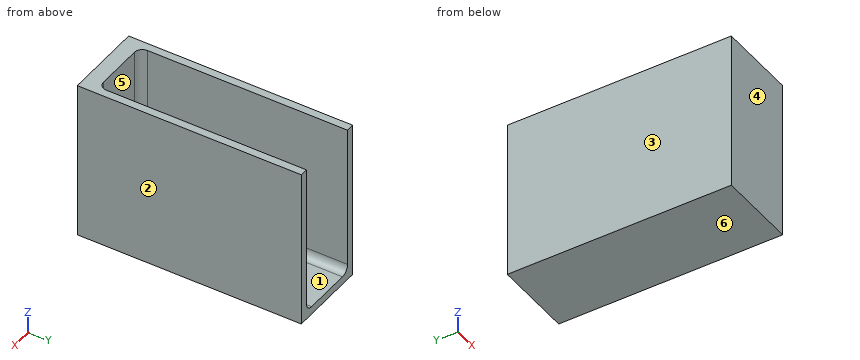
```python
from build123d import *

# Parameters (mm, degrees)
SKETCH1_W           = 25.4
SKETCH1_H           = 50.8
BOSS_EXTRUDE1_DEPTH = 5.08
BOSS_EXTRUDE2_DEPTH = 66.04
FILLET1_R           = 2.54


with BuildPart() as part:
    # Sketch1 → Boss-Extrude1 (new body)
    with BuildSketch(Plane(origin=(0, 0, 0), x_dir=(1, 0, 0), z_dir=(0, 1, 0))):
        Rectangle(SKETCH1_W, SKETCH1_H)
    extrude(amount=BOSS_EXTRUDE1_DEPTH)

    # Sketch2 → Boss-Extrude2 (add)
    with BuildSketch(Plane(origin=(0, 5.08, 0), x_dir=(1, 0, 0), z_dir=(0, 1, 0))):
        Polygon((-12.7, -25.4), (-12.7, 25.4), (12.7, 25.4), (12.7, -25.4), (10.16, -25.4), (10.16, 22.86), (-10.16, 22.86), (-10.16, -25.4), align=None)
    extrude(amount=BOSS_EXTRUDE2_DEPTH)

    # Fillet1
    fillet1_edges = [part.edges().sort_by_distance(p)[0] for p in [
        (-10.16, 5.08, 1.27),
        (0, 5.08, -22.86),
        (-10.16, 38.1, -22.86),
        (10.16, 5.08, 1.27),
        (10.16, 38.1, -22.86),
    ]]
    fillet(fillet1_edges, radius=FILLET1_R)


solid = part.part
```
Verification items for the finished model (mm, model axes). Face numbers are marked on the shaded views. A direction names the side the tool comes from. Coordinates: 2 decimals unless noted, no trailing zeros. Write each loop counter-clockwise with the first axis right and the second up, starting at its lowest first coordinate (ties: lowest second). Pieces come first, ordered by that corner, then holes. Notation, with made-up numbers: M 29,45.5 L 72,45.5 A24 ccw 72,74.5 Z; hole C 3,21 d7. An arc over 180 degrees is marked long. Answer as a JSON object with one key per item and string values. Group by question number.
(1) Tool access check on the marked faces 5 and 6. Record the directions out of +Z, -Z, +X, -X, +Y, -Y that give a thin tool (end or side, any length) a straight path to the whole face; none if there is none.
(2) Cross-section at A-A, the plane y = 54. Record the cut outline in (x, z), and give its area (3 significant figures).
(3) Release check for a two-part mould opening along X. For the marked faces 1, 2, 3 and 4 record: +X half, -X half, draft (parallel to the pull), parting line (faces both ways), or undercut.
(4) Cross-section at B-B, the plane z = 15. Record the cut outline in (x, y), and give its area (3 significant figures).
(5) Gauge pin test, flat ends, axial feed: pin 1 (6 mm diameter, centred on x = -5.5, z = -15, fed in from +Y); pin 2 (1.5 mm diameter, centred on x = -2, y = 40, fed in from +Z); pin 3 (1.5 mm diameter, centred on x = 5.5, z = 8.5, fed in from +Y). Record the tip position at first contact, or that the pin passes through.
(6) Cross-section at C-C, the plane x = -5.5. Record the cut outline in (y, z).
(7) Material ranges on line 1 (X direction, y = 31.5, z = -5.5); line 2 (Z direction, x = 6.5, y = 45); line 3 (Y direction, x = 0, z = 8), recorded low to high.
Reply:
{
 "1": {"face 5": "+Z, +Y", "face 6": "-Z, +X, -X, +Y, -Y"},
 "2": {"outline": "M -12.7,-25.4 L 12.7,-25.4 L 12.7,25.4 L 10.16,25.4 L 10.16,-20.32 A2.54 cw 7.62,-22.86 L -7.62,-22.86 A2.54 cw -10.16,-20.32 L -10.16,25.4 L -12.7,25.4 Z", "area": "312 mm²"},
 "3": {"face 1": "undercut", "face 2": "+X half", "face 3": "-X half", "face 4": "draft"},
 "4": {"outline": "M -12.7,0 L 12.7,0 L 12.7,71.12 L 10.16,71.12 L 10.16,7.62 A2.54 cw 7.62,5.08 L -7.62,5.08 A2.54 cw -10.16,7.62 L -10.16,71.12 L -12.7,71.12 Z", "area": "467 mm²"},
 "5": {"pin 1": "y = 5.24", "pin 2": "z = -22.86", "pin 3": "y = 5.08"},
 "6": {"outline": "M 0,-25.4 L 71.12,-25.4 L 71.12,-22.86 L 7.62,-22.86 A2.54 cw 5.08,-20.32 L 5.08,25.4 L 0,25.4 Z"},
 "7": {"line 1": "-12.7 to -10.16, 10.16 to 12.7", "line 2": "-25.4 to -22.86", "line 3": "0 to 5.08"}
}
